Verification items for this drawing (mm, ordinates from the low corner). Give positions to 0.01 mm unless a question says otherwise; leave off trailing zeros. Loops run counter-clockwise (first coordinate to the right, second up) from the corner with the lowest first, then second, coordinate; pieces in that order, holes last. Notation, with made-up numbers: M 10.5,29.5 L 21.5,29.5 A35 cw 21.5,61.5 Z; hole C 82.25,26.25 d10. An arc over 180 degrees is marked long. Use a Markdown table: item, result.
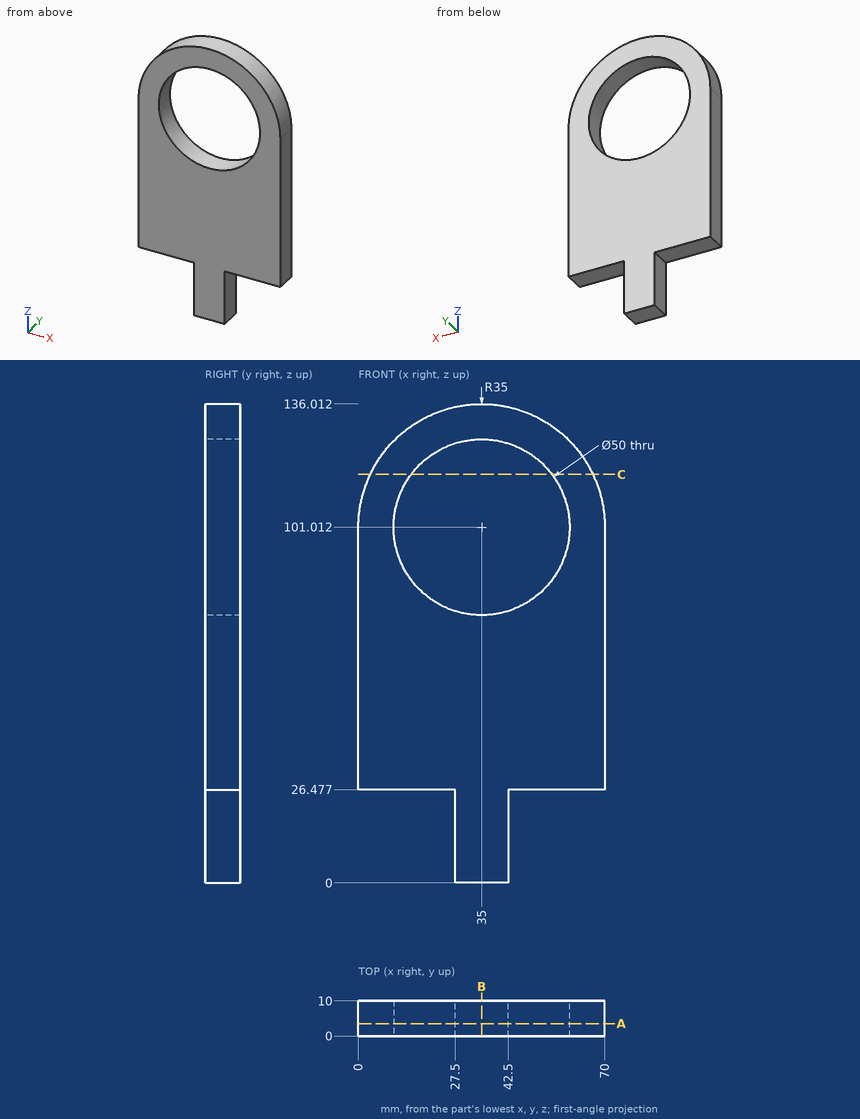
(1) Material ranges on line 1 (Z direction, x = 35, y = 6.5); line 2 (X direction, y = 2.5, z = 108) (1 decimal); line 3 (X direction, y = 6, z = 111.5), recorded low to high.
Results below:
| item | result |
|---|---|
| line 1 | 0 to 76.01, 126.01 to 136.01 |
| line 2 | 0.7 to 11, 59 to 69.3 |
| line 3 | 1.61 to 12.31, 57.69 to 68.39 |
(2) Cross-section at B-B on x = 35. Record the cut outline in (y, z), then the cut area to 3 significant figures.
Results below:
| item | result |
|---|---|
| outline | M 0,0 L 10,0 L 10,76.01 L 0,76.01 Z; M 0,126.01 L 10,126.01 L 10,136.01 L 0,136.01 Z |
| area | 860 mm^2 |
(3) Gauge pin test, flat ends, axial feed: P1, Ø2, axis at y = 3.5, z = 103.5, coming from the -X side; P2, Ø2, axis at y = 8, z = 114, coming from the +X side; P3, Ø3, axis at y = 4, z = 122.5, coming from the -X side; P4, Ø5, axis at x = 48.5, z = 59, coming from the -Y side. Record the tip position at first contact, or that the pin passes through.
Results below:
| item | result |
|---|---|
| P1 | x = 0.03 |
| P2 | x = 67.88 |
| P3 | x = 6.27 |
| P4 | y = 0 |
(4) Cross-section at C-C on z = 116. Record the cut outline in (x, y).
Results below:
| item | result |
|---|---|
| outline | M 3.37,0 L 14.99,0 L 14.99,10 L 3.37,10 Z; M 55.01,0 L 66.63,0 L 66.63,10 L 55.01,10 Z |
(5) Cross-section at A-A on y = 3.5. Record the cut outline in (x, z).
Results below:
| item | result |
|---|---|
| outline | M 0,26.48 L 27.5,26.48 L 27.5,0 L 42.5,0 L 42.5,26.48 L 70,26.48 L 70,101.01 A35 ccw 0,101.01 Z; hole C 35,101.01 d50 |
